Design review of the part built by this model. Coordinates are the model's own, in mm. A direction names the side the tool comes from. Coordinates: 2 decimals unless noted, no trailing zeros. Loops run counter-clockwise (first coordinate to the right, second up) from the corner with the lowest first, then second, coordinate; pieces in that order, holes last. Notation, with made-up numbers: (2.25, -35.5) - (44.25, -35.5) arc R26 ccw to (44.25, 2.5) - close; hole circle Ø2 at (-24, 11). An arc over 180 degrees is marked (long way). Answer in a Markdown table with one row per item. Add a question column.
(1) Clearance check with flat-ended pins moving along their axes: pin 1 (0.6 mm diameter, centred on x = -64, y = -6, fed in from -Z); pin 2 (1 mm diameter, centred on x = -41.5, y = -0.5, fed in from +Z); pin 3 (2.5 mm diameter, centred on x = -36, y = -3.5, fed in from +Z). State where each tip first meets the part, or that it passes through.
(2) The part is to be moulded in two halves that separate along X. For faces 6 (the face through (-65, -3, 68.326)), 7 (the face through (-25, -3, -9.523)), 8 (the face through (18.121, -2, 33)), 9 (the face through (-24, -3, 42.393)), say which applies: released by +X, released by -X, zero draft, split by the parting line, or undercut.
(3) We need section A-A, the plane z = 24. Write out the cut boundary in (x, y), plus the area to 3 significant figures.
(4) To check wall thickness, follow L1, parallel to X at y = -1.5, z = -24.5; L2, parallel to Z at x = -25.5, y = -0.75; L3, parallel to Z at x = -28.5, y = -1.5. State the ranges of each line that lie inside material, in increasing order. Write a range as [from, to].
(5) We need section C-C, the plane x = -69.5. Write out the cut boundary in (y, z).
(6) We need section B-B, the plane y = -1.75. Give the number of separate pieces and of enclosed holes in the cut face, plus the area to 3 significant figures.
(7) For faces 1 (the face through (-61.381, -3, 46)), 2 (the face through (-76, -3, 46.11)), 3 (the face through (-65, -6.35, 67)), 4 (the face through (-15, -5.08, 42)), 5 (the face through (-61.381, -2, 63)), list the 3-axis set-ups (+Z, -Z, +X, -X, +Y, -Y) from which the entire face can be reached by the end or side of a thin tool; tool diameter is ignored.
from build123d import *

# Parameters (mm, degrees)
F0_W     = 1.524
F0_H     = 2.54
F0_W_2   = 18.542
F0_W_3   = 53.086
F1_DEPTH = 5.08
F0_W_4   = 6.35
F0_W_5   = 15.748
F0_H_2   = 3.1443536282
F2_DEPTH = 6.35
F0_H_3   = 9.6294713412
F0_H_4   = 65.7186827598
F3_DEPTH = 6.096
F4_DEPTH = 5.08
F5_DEPTH = 5.08
F6_DEPTH = 5.08


with BuildPart() as f1:
    # F0 (on Front) → F1 (new body)
    with BuildSketch(Plane.XZ):
        with BuildLine():
            add(Edge.make_bspline(
                [(-61.3806553816, 58.2051597101), (-43.8441733015, 55.3503870336), (-19.0644229117, 65.9568732466), (0, 81.5450566713), (11.7713446184, 75.4133064361)],
                knots=[0, 0, 0, 0, 0.5425588266, 1, 1, 1, 1], degree=3))
            Line((-61.3806553816, 58.2051597101), (-61.3806553816, 50.5851597101))
            add(Edge.make_bspline(
                [(-61.3806553816, 50.5851597101), (-54.5700391068, 50.2481911872), (-48.4601444481, 50.6597637989), (-42.8386553816, 51.696558085)],
                knots=[0, 0, 0, 0, 0.2106262028, 0.2106262028, 0.2106262028, 0.2106262028], degree=3))
            add(Edge.make_bspline(
                [(-42.8386553816, 51.696558085), (-42.3266573649, 51.7909879792), (-41.8187108352, 51.8906042954), (-41.3146553816, 51.9953138621)],
                knots=[0.2106262028, 0.2106262028, 0.2106262028, 0.2106262028, 0.2298097673, 0.2298097673, 0.2298097673, 0.2298097673], degree=3))
            add(Edge.make_bspline(
                [(-41.3146553816, 51.9953138621), (-33.2393780699, 53.6728252996), (-15.5050873091, 61.1527435678), (0.0995686219, 74.4364412814), (11.7713446184, 67.7933064361)],
                knots=[0.2298097673, 0.2298097673, 0.2298097673, 0.2298097673, 0.5371422287, 1, 1, 1, 1], degree=3))
            Line((11.7713446184, 67.7933064361), (11.7713446184, 75.4133064361))
        make_face()
        Polygon((-67.7306553816, 65.7861350714), (-67.7306553816, 46.1095218752), (-67.7306553816, 36.480050534), (-67.7306553816, 33.3356969059), (-67.7306553816, -32.382985854), (-61.3806553816, -32.382985854), (-61.3806553816, -26.2942135113), (-61.3806553816, -9.522985854), (-61.3806553816, -6.982985854), (-61.3806553816, -1.905), (-61.3806553816, -0.9525), (-61.3806553816, 0), (-61.3806553816, 10.16), (-61.3806553816, 11.1125), (-61.3806553816, 12.065), (-61.3806553816, 20.997421816), (-61.3806553816, 22.267421816), (-61.3806553816, 39.8533064361), (-61.3806553816, 42.3933064361), (-61.3806553816, 42.9651597101), (-61.3806553816, 50.5851597101), (-61.3806553816, 58.2051597101), (-61.3806553816, 65.7861350714), align=None)
        Polygon((-61.3806553816, -26.2942135113), (-61.3806553816, -32.382985854), (11.7713446184, -32.382985854), (11.7713446184, -26.2942135113), (-41.3146553816, -26.2942135113), (-42.8386553816, -26.2942135113), align=None)
        Polygon((11.7713446184, 97.157014146), (11.7713446184, 75.4133064361), (11.7713446184, 67.7933064361), (11.7713446184, 46.1095218752), (11.7713446184, 42.3933064361), (11.7713446184, 39.8533064361), (11.7713446184, 22.267421816), (11.7713446184, 20.997421816), (11.7713446184, 19.2415746087), (11.7713446184, 17.9715746087), (11.7713446184, 12.065), (11.7713446184, 11.1125), (11.7713446184, 10.16), (11.7713446184, 0), (11.7713446184, -0.9525), (11.7713446184, -1.905), (11.7713446184, -6.982985854), (11.7713446184, -9.522985854), (11.7713446184, -26.2942135113), (11.7713446184, -32.382985854), (18.1213446184, -32.382985854), (18.1213446184, 97.157014146), align=None)
        with Locations((-42.0766553816, -8.252985854)):
            Rectangle(F0_W, F0_H)
        with Locations((-52.1096553816, -8.252985854)):
            Rectangle(F0_W_2, F0_H)
        with Locations((-14.7716553816, -8.252985854)):
            Rectangle(F0_W_3, F0_H)
        with Locations((-14.7716553816, 41.1233064361)):
            Rectangle(F0_W_3, F0_H)
        with Locations((-52.1096553816, 41.1233064361)):
            Rectangle(F0_W_2, F0_H)
        with Locations((-42.0766553816, 41.1233064361)):
            Rectangle(F0_W, F0_H)
    extrude(amount=F1_DEPTH)

    # F0 (on Front) → F2 (join)
    with BuildSketch(Plane.XZ):
        with Locations((-64.5556553816, 67.0561350714)):
            Rectangle(F0_W_4, F0_H)
        with Locations((14.9463446184, 98.427014146)):
            Rectangle(F0_W_4, F0_H)
        with Locations((-75.6046553816, 34.9078737199)):
            Rectangle(F0_W_5, F0_H_2)
    extrude(amount=F2_DEPTH)

    # F0 (on Front) → F3 (join)
    with BuildSketch(Plane.XZ):
        with Locations((-75.6046553816, 41.2947862046)):
            Rectangle(F0_W_5, F0_H_3)
        with Locations((-75.6046553816, 0.4763555259)):
            Rectangle(F0_W_5, F0_H_4)
    extrude(amount=F3_DEPTH)

    # F0 (on Front) → F4 (cut)
    with BuildSketch(Plane.XZ):
        with Locations((-52.1096553816, 41.1233064361)):
            Rectangle(F0_W_2, F0_H)
        with Locations((-42.0766553816, 41.1233064361)):
            Rectangle(F0_W, F0_H)
        with Locations((-14.7716553816, 41.1233064361)):
            Rectangle(F0_W_3, F0_H)
    extrude(amount=F4_DEPTH, mode=Mode.SUBTRACT)

    # F0 (on Front) → F5 (cut)
    with BuildSketch(Plane.XZ):
        with Locations((-52.1096553816, -8.252985854)):
            Rectangle(F0_W_2, F0_H)
        with Locations((-42.0766553816, -8.252985854)):
            Rectangle(F0_W, F0_H)
        with Locations((-14.7716553816, -8.252985854)):
            Rectangle(F0_W_3, F0_H)
    extrude(amount=F5_DEPTH, mode=Mode.SUBTRACT)

    # F0 (on Front) → F6 (join)
    with BuildSketch(Plane.XZ):
        with Locations((-14.7716553816, 41.1233064361)):
            Rectangle(F0_W_3, F0_H)
        with Locations((-52.1096553816, 41.1233064361)):
            Rectangle(F0_W_2, F0_H)
        with Locations((-42.0766553816, 41.1233064361)):
            Rectangle(F0_W, F0_H)
        with Locations((-52.1096553816, -8.252985854)):
            Rectangle(F0_W_2, F0_H)
        with Locations((-14.7716553816, -8.252985854)):
            Rectangle(F0_W_3, F0_H)
        with Locations((-42.0766553816, -8.252985854)):
            Rectangle(F0_W, F0_H)
    extrude(amount=F6_DEPTH)


solid = f1.part
Responses:
| question | item | result |
|---|---|---|
| 1 | pin 1 | stops at z = 65.79 |
| 1 | pin 2 | stops at z = 58.69 |
| 1 | pin 3 | stops at z = 60.46 |
| 2 | face 6 | zero draft |
| 2 | face 7 | undercut |
| 2 | face 8 | released by +X |
| 2 | face 9 | undercut |
| 3 | outline | (-83.48, -6.1) - (-67.73, -6.1) - (-67.73, -5.08) - (-61.38, -5.08) - (-61.38, 0) - (-83.48, 0) - close; (11.77, -5.08) - (18.12, -5.08) - (18.12, 0) - (11.77, 0) - close |
| 3 | area | 161 mm2 |
| 4 | L1 | x = [-83.48, -61.38], [11.77, 18.12] |
| 4 | L2 | z = [-32.38, -26.29], [-9.52, -6.98], [39.85, 42.39], [57.36, 64.44] |
| 4 | L3 | z = [-32.38, -26.29], [-9.52, -6.98], [39.85, 42.39], [56.01, 62.98] |
| 5 | outline | (-6.35, 33.34) - (-6.1, 33.34) - (-6.1, -32.38) - (0, -32.38) - (0, 46.11) - (-6.1, 46.11) - (-6.1, 36.48) - (-6.35, 36.48) - close |
| 6 | separate pieces | 1 |
| 6 | enclosed holes | 3 |
| 6 | area | 4,050 mm2 |
| 7 | face 1 | +Y, -Y |
| 7 | face 2 | +Z, -X, +Y, -Y |
| 7 | face 3 | +Z, -Z, +X, -X, -Y |
| 7 | face 4 | -Z, +X, -Y |
| 7 | face 5 | +Z, +Y, -Y |
